Autodesk Inventor part; units mm, degrees
ref_plane "YZ Plane" through (0, 0, 0) normal (1, 0, 0) x (0, 1, 0)
ref_plane "XZ Plane" through (0, 0, 0) normal (0, 1, 0) x (-1, 0, 0)
ref_plane "XY Plane" through (0, 0, 0) normal (0, 0, 1) x (1, 0, 0)
sketch "Sketch2" plane through (0, 0, 0) normal (0, 1, 0) x (-1, 0, 0)
  circle A0 centre (0, 0) radius 18.75
  circle A1 centre (0, 0) radius 30
  circle A2 centre (26, 0) radius 1.6
  circle A3 centre (18.3848, -18.3848) radius 1.6
  circle A4 centre (0, -26) radius 1.6
  circle A5 centre (-18.3848, -18.3848) radius 1.6
  circle A6 centre (-26, 0) radius 1.6
  circle A7 centre (-18.3848, 18.3848) radius 1.6
  circle A8 centre (0, 26) radius 1.6
  circle A9 centre (18.3848, 18.3848) radius 1.6
  dimension "motorDiameter" = 37.5
  dimension "motorFixtureDiameter" = 60
  dimension "d20" = 3.2
  dimension "d21" = 26
  dimension "d24" = 0
  dimension "d27" = 360
extrude "Extrusion2" add sketch "Sketch2" along normal blind 2.5
sketch "Sketch3" plane through (0, 2.5, 0) normal (0, 1, 0) x (1, 0, 0)
  circle A0 centre (2, 0) radius 21.15
  circle A1 centre (0, 0) radius 18.75
  dimension "d31" = 2
  dimension "d32" = 42.3
  dimension "d33" = 37.5
  dimension "d34" = 0
extrude "Extrusion3" add sketch "Sketch3" along normal blind 20
sketch "Sketch4" plane through (2, 22.5, 0) normal (0, 1, 0) x (1, 0, 0)
  circle A0 centre (0, 0) radius 21.15
  circle A1 centre (0, 0) radius 21.15
extrude "Extrusion4" add sketch "Sketch4" along normal blind 6
sketch "Sketch5" plane through (2, 28.5, 0) normal (0, 1, 0) x (1, 0, 0)
  circle A0 centre (-2, 0) radius 18.75
  circle A1 centre (0, 0) radius 21.15
  circle A2 centre (0, 0) radius 21.15
  circle A3 centre (5, 0) radius 6.25
  circle A4 centre (-2, 15.5) radius 1.6
  circle A5 centre (-15.4234, 7.75) radius 1.6
  circle A6 centre (-15.4234, -7.75) radius 1.6
  circle A7 centre (-2, -15.5) radius 1.6
  circle A8 centre (11.4234, -7.75) radius 1.6
  circle A9 centre (11.4234, 7.75) radius 1.6
  dimension "d39" = 12.5
  dimension "d40" = 0
  dimension "d43" = 3.2
  dimension "d44" = 0
  dimension "d45" = 15.5
  dimension "d48" = 360
  dimension "d52" = 7
extrude "Extrusion5" cut sketch "Sketch5" against normal up to next contours A3 | A4 | A5 | A6 | A7 | A8 | A9
equation "\"d33\" = motorDiameter"
properties part number "motor fixture" material "ABS Plastic"
Design review of the part built by this model. Coordinates are the model's own, in mm. A direction names the side the tool comes from. Round coordinates to 2 decimals unless told otherwise and drop trailing zeros. Write each loop counter-clockwise with the first axis right and the second up, starting at its lowest first coordinate (ties: lowest second). Pieces come first, ordered by that corner, then holes. Notation, with made-up numbers: M 82.5,19 L 114.5,19 A19 ccw 114.5,51 Z; hole C 29.25,17 d6. An arc over 180 degrees is marked long. One line per item, written item: value. Start each with the question number.
1. Take a section at C-C on z = -26. State the section outline as (x, y) points, then the cut area to 3 significant figures.
2. Take a section at A-A on y = 24.5. State the section outline as (x, z) points, then the cut area to 3 significant figures.
3. Draft analysis for pull direction Z (two halves, no side actions). For faces 4 (the face through (29.97, 1.23, -1.32)), 5 (the face through (2, 28.5, 4)), 6 (the face through (0.756, 25.542, -0.275)), state which applies: pulls with the +Z half, pulls with the -Z half, needs draft (parallel to the pull), parting line crosses it, or undercut.
4. For faces 1 (the face through (-20, 2.5, 0)), 2 (the face through (1.24, 11.09, 18.71)), 3 (the face through (0.208, 1.232, 24.414)), list the 3-axis set-ups (+Z, -Z, +X, -X, +Y, -Y) from which the entire face can be reached by the end or side of a thin tool; tool diameter is ignored.
5. Take a section at D-D on x = 26. State the section outline as (y, z) points, then the cut area to 3 significant figures.
6. To check wall thickness, follow probe 1 along Z at (x, y) = (0, 0.6); probe 2 along Z at (x, y) = (0, 24.2); probe 3 along Y at (x, z) = (9.5, 15.5). State the ranges of each line that lie inside material, in increasing order. Write a range as from..to.
7. Clearance check with flat-ended pins moving along their axes: P1, Ø3, axis at x = -18.38, z = -18.38, coming from the +Y side; P2, Ø1, axis at y = 22, z = -2, coming from the +X side; P3, Ø8, axis at y = 5.5, z = 21, coming from the -X side; P4, Ø6, axis at x = -18, y = 14.5, coming from the -Z side. State where each tip first meets the part, or that it passes through.
Computed:
1. outline: M -14.97,0 L -1.6,0 L -1.6,2.5 L -14.97,2.5 Z; M 1.6,0 L 14.97,0 L 14.97,2.5 L 1.6,2.5 Z
1. area: 66.8 mm²
2. outline: C 2,0 d42.3; hole C -13.42,-7.75 d3.2; hole C -13.42,7.75 d3.2; hole C 0,-15.5 d3.2; hole C 0,15.5 d3.2; hole C 7,0 d12.5; hole C 13.42,-7.75 d3.2; hole C 13.42,7.75 d3.2
2. area: 1,230 mm²
3. face 4: parting line crosses it
3. face 5: needs draft
3. face 6: undercut
4. face 1: +Y
4. face 2: -Y
4. face 3: +Y, -Y
5. outline: M 0,-14.97 L 2.5,-14.97 L 2.5,-1.6 L 0,-1.6 Z; M 0,1.6 L 2.5,1.6 L 2.5,14.97 L 0,14.97 Z
5. area: 66.8 mm²
6. probe 1: z = -30..-27.6, -24.4..-18.75, 18.75..24.4, 27.6..30
6. probe 2: z = -21.06..-17.1, -13.9..13.9, 17.1..21.06
6. probe 3: y = 22.5..28.5
7. P1: passes through
7. P2: stops at x = 23.1
7. P3: stops at x = -23.73
7. P4: stops at z = -12.58
